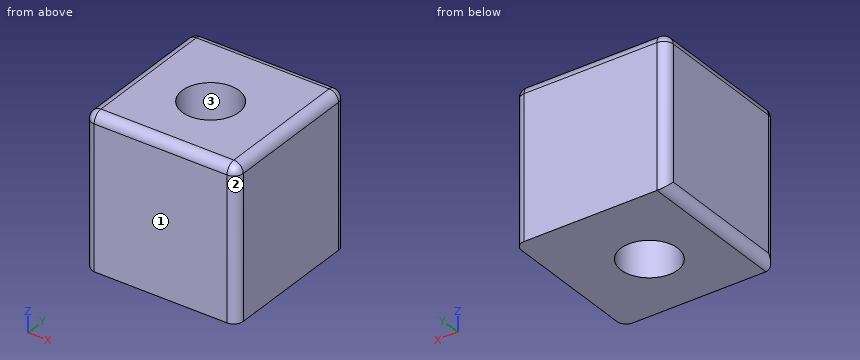
```python
from build123d import *

# Parameters (mm, degrees)
F0_W     = 80
F0_H     = 80
F1_DEPTH = 80
F2_R     = 15
F3_DEPTH = 80.001
F4_R     = 5


with BuildPart() as f1:
    # F0 (on Top) → F1 (new body)
    with BuildSketch(Plane.XY):
        with Locations((-19.29054, 2.671687)):
            Rectangle(F0_W, F0_H)
    extrude(amount=F1_DEPTH)

    # F2 (on face) → F3 (cut, through all)
    with BuildSketch(Plane.XY.offset(80)):
        with Locations((-19.669065, 0)):
            Circle(F2_R)
    extrude(amount=-F3_DEPTH, mode=Mode.SUBTRACT)

    # F4
    f4_edges = [f1.edges().sort_by_distance(p)[0] for p in [
        (-19.29054, 42.671687, 80),
        (-59.29054, 2.671687, 80),
        (-19.29054, -37.328313, 80),
        (-59.29054, 42.671687, 40),
        (-59.29054, -37.328313, 40),
        (-59.29054, 2.671687, 0),
        (20.70946, 42.671687, 40),
        (20.70946, -37.328313, 40),
        (20.70946, 2.671687, 80),
    ]]
    fillet(f4_edges, radius=F4_R)


solid = f1.part
```
CAD build for the part. Positions are in the model's coordinates, mm. Face numbers are marked on the shaded views. Coordinates: 2 decimals unless noted, no trailing zeros. Write each loop counter-clockwise with the first axis right and the second up, starting at its lowest first coordinate (ties: lowest second). Pieces come first, ordered by that corner, then holes.
(1) Cut at B-B, the plane z = 38. List the corners of the cut face in (x, y).
(2) Cut at D-D, the plane y = -12. List the corners of the cut face in (x, z).
(3) Drill centre lines: probe 1 along Y at (x, z) = (-19.5, 25.5); probe 2 along Y at (x, z) = (-23.5, 25); probe 3 along X at (y, z) = (11, 38.5). Where is each one in solid material? Low to high.
(4) Two-plate mould, pull along X, no slides. Class the marked faces 1, 2 and 3: +X half, -X half, draft (parallel to the pull), parting line (faces both ways), or undercut.
(5) Cut at C-C, the plane x = -14. List the corners of the cut face in (y, z), and give its area (3 significant figures).
(6) Cut at A-A, the plane y = 0. List the corners of the cut face in (x, z).
Geometry says:
1. outline: (-59.29, -32.33) arc R5 ccw to (-54.29, -37.33) - (15.71, -37.33) arc R5 ccw to (20.71, -32.33) - (20.71, 37.67) arc R5 ccw to (15.71, 42.67) - (-54.29, 42.67) arc R5 ccw to (-59.29, 37.67) - close; hole circle Ø30 at (-19.67, 0)
2. outline: (-59.29, 5) arc R5 ccw to (-54.29, 0) - (-28.67, 0) - (-28.67, 80) - (-54.29, 80) arc R5 ccw to (-59.29, 75) - close; (-10.67, 0) - (20.71, 0) - (20.71, 75) arc R5 ccw to (15.71, 80) - (-10.67, 80) - close
3. probe 1: y = -37.33 to -15, 15 to 42.67
3. probe 2: y = -37.33 to -14.5, 14.5 to 42.67
3. probe 3: x = -59.29 to -29.87, -9.47 to 20.71
4. face 1: draft
4. face 2: +X half
4. face 3: undercut
5. outline: (-37.33, 0) - (-13.89, 0) - (-13.89, 80) - (-32.33, 80) arc R5 ccw to (-37.33, 75) - close; (13.89, 0) - (42.67, 0) - (42.67, 75) arc R5 ccw to (37.67, 80) - (13.89, 80) - close
5. area: 4,170 mm2
6. outline: (-59.29, 5) arc R5 ccw to (-54.29, 0) - (-34.67, 0) - (-34.67, 80) - (-54.29, 80) arc R5 ccw to (-59.29, 75) - close; (-4.67, 0) - (20.71, 0) - (20.71, 75) arc R5 ccw to (15.71, 80) - (-4.67, 80) - close
